```python
from build123d import *

# Parameters (mm, degrees)
SKETCH2_R           = 2.15
BOSS_EXTRUDE1_DEPTH = 100
CUT_EXTRUDE1_DEPTH  = 21
CUT_EXTRUDE2_DEPTH  = 21


with BuildPart() as part:
    # Sketch2 → Boss-Extrude1 (new body, symmetric)
    with BuildSketch(Plane.XY):
        Polygon((-2.5, 10), (-2.5, 8.2), (-6.927207794, 8.2), (-2.677207794, 3.95), (2.677207794, 3.95), (6.927207794, 8.2), (2.5, 8.2), (2.5, 10), (10, 10), (10, 2.5), (8.2, 2.5), (8.2, 6.927207794), (3.95, 2.677207794), (3.95, -2.677207794), (8.2, -6.927207794), (8.2, -2.5), (10, -2.5), (10, -10), (2.5, -10), (2.5, -8.2), (6.927207794, -8.2), (2.677207794, -3.95), (-2.677207794, -3.95), (-6.927207794, -8.2), (-2.5, -8.2), (-2.5, -10), (-10, -10), (-10, -2.5), (-8.2, -2.5), (-8.2, -6.927207794), (-3.95, -2.677207794), (-3.95, 2.677207794), (-8.2, 6.927207794), (-8.2, 2.5), (-10, 2.5), (-10, 10), align=None)
        Circle(SKETCH2_R, mode=Mode.SUBTRACT)
    extrude(amount=BOSS_EXTRUDE1_DEPTH, both=True)

    # Sketch3 → Cut-Extrude1 (cut, through all)
    with BuildSketch(Plane(origin=(0, 10, 0), x_dir=(1, 0, 0), z_dir=(0, 1, 0))):
        Polygon((-10, -100), (10, -100), (-10, -92.720595315), align=None)
    extrude(amount=-CUT_EXTRUDE1_DEPTH, mode=Mode.SUBTRACT)

    # Sketch4 → Cut-Extrude2 (cut, through all)
    with BuildSketch(Plane(origin=(0, 10, 0), x_dir=(1, 0, 0), z_dir=(0, 1, 0))):
        Polygon((10, 100), (-10, 100), (-10, 92.720595315), align=None)
    extrude(amount=-CUT_EXTRUDE2_DEPTH, mode=Mode.SUBTRACT)


solid = part.part
```
CAD build for the part. Positions are in the model's coordinates, mm. Coordinates: 2 decimals unless noted, no trailing zeros. Loops run counter-clockwise (first coordinate to the right, second up) from the corner with the lowest first, then second, coordinate; pieces in that order, holes last. Notation, with made-up numbers: (0, -36) - (43, -36) arc R18 ccw to (43, -21) - close; hole circle Ø11 at (48, -15.75). An arc over 180 degrees is marked (long way). Use CSV: the item, a comma, the result in double quotes. Start each with the question number.
Q1. Two-plate mould, pull along X, no slides. Class faces 1 (the flat face through (0.14, 2.36, 96.41)), 2 (the flat face through (-6, 10, 1)), 3 (the flat face through (8.2, 5, 1)): +X half, -X half, draft (parallel to the pull), parting line (faces both ways), or undercut.
Q2. Cut at B-B, the plane y = 0. List the corners of the cut face in (x, z).
Q3. Drop flat-ended pins along their axis: P1, Ø2.5, axis at y = 0.5, z = -2.5, coming from the +X side; P2, Ø8, axis at x = -5.5, y = 3, coming from the +Z side; P3, Ø8, axis at x = -0.5, y = -0.5, coming from the +Z side; P4, Ø2, axis at x = -0.5, y = 5.5, coming from the +Z side. Give the stop position or say it passes through.
Q4. Cut at A-A, the plane x = -0.5. List the corners of the cut face in (y, z).
Q5. Probe probe 1 along X at (y, z) = (0, 41.5); probe 2 along Y at (x, z) = (3.5, 84.5). List the from-to ranges inside material, lowest first. Write a range as from..to.
Here are the results:
1,face 1,"-X half"
1,face 2,"draft"
1,face 3,"undercut"
2,outline,"(-3.95, -94.92) - (-2.15, -95.58) - (-2.15, 95.58) - (-3.95, 94.92) - close; (2.15, -97.14) - (3.95, -97.8) - (3.95, 97.8) - (2.15, 97.14) - close"
3,P1,"x = 3.95"
3,P2,"z = 95.81"
3,P3,"z = 97.63"
3,P4,"through"
4,outline,"(-3.95, -96.18) - (-2.09, -96.18) - (-2.09, 96.18) - (-3.95, 96.18) - close; (2.09, -96.18) - (3.95, -96.18) - (3.95, 96.18) - (2.09, 96.18) - close"
5,probe 1,"-3.95..-2.15, 2.15..3.95"
5,probe 2,"-10..-8.2, -4.77..4.77, 8.2..10"
